For this review, take the finished solid that the model builds, in its own axes (mm). Face numbers are marked on the shaded views. A direction names the side the tool comes from. Give positions to 0.01 mm unless a question says otherwise; leave off trailing zeros. Loops run counter-clockwise (first coordinate to the right, second up) from the corner with the lowest first, then second, coordinate; pieces in that order, holes last. Notation, with made-up numbers: (17.25, 3) - (51.25, 3) arc R24 cw to (51.25, 39) - close; hole circle Ø8 at (42, -18.75). An arc over 180 degrees is marked (long way). Answer in a Markdown table with one row per item.
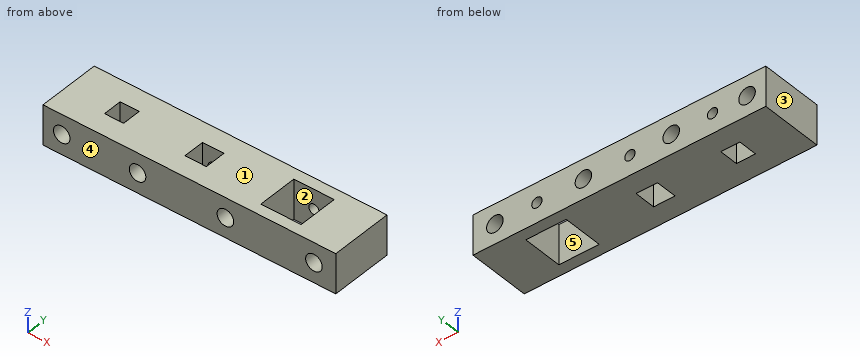
```python
from build123d import *

# Parameters (mm, degrees)
SKETCH1_W                       = 93.728
SKETCH1_H                       = 20
SKETCH1_W_2                     = 6.1
SKETCH1_H_2                     = 6.1
SKETCH1_W_3                     = 6.858
SKETCH1_H_3                     = 6.858
SKETCH1_W_4                     = 12.9
SKETCH1_H_4                     = 12.9
BOSS_EXTRUDE1_DEPTH             = 12.7
TAP_DRILL_FOR_M4X0_7_TAP1_D     = 3.3
TAP_DRILL_FOR_M4X0_7_TAP1_DEPTH = 6.95
M5_CLEARANCE_HOLE1_D            = 5.3


with BuildPart() as part:
    # Sketch1 → Boss-Extrude1 (new body)
    with BuildSketch(Plane.XY):
        with Locations((3.375, 0)):
            Rectangle(SKETCH1_W, SKETCH1_H)
        with Locations((-26.439, 0)):
            Rectangle(SKETCH1_W_2, SKETCH1_H_2, mode=Mode.SUBTRACT)
        Rectangle(SKETCH1_W_3, SKETCH1_H_3, mode=Mode.SUBTRACT)
        with Locations((29.789, 0)):
            Rectangle(SKETCH1_W_4, SKETCH1_H_4, mode=Mode.SUBTRACT)
    extrude(amount=BOSS_EXTRUDE1_DEPTH)

    # Tap Drill for M4x0.7 Tap1
    with Locations(Plane(origin=(-26.439, 10, 6.35), x_dir=(0, 0, 1), z_dir=(0, 1, 0))):
        with Locations((0, 0), (0, 26.439), (0, 56.228)):
            Hole(TAP_DRILL_FOR_M4X0_7_TAP1_D / 2, depth=TAP_DRILL_FOR_M4X0_7_TAP1_DEPTH)

    # M5 Clearance Hole1 (through all)
    with Locations(Plane(origin=(-37.489, 10, 6.35), x_dir=(0, 0, 1), z_dir=(0, 1, 0))):
        with Locations((0, 0), (0, 24.2695), (0, 52.3835), (0, 80.728)):
            Hole(M5_CLEARANCE_HOLE1_D / 2)


solid = part.part
```
1. For the marked faces 4 and 5, list the 3-axis set-ups (+Z, -Z, +X, -X, +Y, -Y) from which the entire face can be reached by the end or side of a thin tool; tool diameter is ignored.
Values:
| item | result |
|---|---|
| face 4 | +Z, -Z, +X, -X, -Y |
| face 5 | +Z, -Z |
2. Clearance check with a flat-ended pin moving along its axis: pin 1 (2.5 mm diameter, centred on x = 0, z = 6.35, fed in from +Y). State where the tip first meets the part, or that it passes through.
Values:
| item | result |
|---|---|
| pin 1 | stops at y = -3.43 |
3. Mouldability with a two-part tool opening along X and no side actions: class the marked faces 1, 2 and 3 as released by +X, released by -X, zero draft, split by the parting line, or undercut.
Values:
| item | result |
|---|---|
| face 1 | zero draft |
| face 2 | undercut |
| face 3 | released by -X |
4. We need section C-C, the plane y = -0.25. Give the boundary of the cut face in (x, z), and give its area (3 significant figures).
Values:
| item | result |
|---|---|
| outline | (-43.49, 0) - (-29.49, 0) - (-29.49, 12.7) - (-43.49, 12.7) - close; (-23.39, 0) - (-3.43, 0) - (-3.43, 12.7) - (-23.39, 12.7) - close; (3.43, 0) - (23.34, 0) - (23.34, 12.7) - (3.43, 12.7) - close; (36.24, 0) - (50.24, 0) - (50.24, 12.7) - (36.24, 12.7) - close; hole circle Ø5.3 at (-37.49, 6.35); hole circle Ø5.3 at (-13.22, 6.35); hole circle Ø5.3 at (14.89, 6.35); hole circle Ø5.3 at (43.24, 6.35) |
| area | 774 mm^2 |
5. We need section A-A, the plane z = 2.5. Give the boundary of the cut face in (x, y), and give its area (3 significant figures).
Values:
| item | result |
|---|---|
| outline | (-43.49, -10) - (50.24, -10) - (50.24, 10) - (-43.49, 10) - close; hole (-29.49, -3.05) - (-23.39, -3.05) - (-23.39, 3.05) - (-29.49, 3.05) - close; hole (-3.43, -3.43) - (3.43, -3.43) - (3.43, 3.43) - (-3.43, 3.43) - close; hole (23.34, -6.45) - (36.24, -6.45) - (36.24, 6.45) - (23.34, 6.45) - close |
| area | 1,620 mm^2 |
6. We need section B-B, the plane x = 44.5. Give the boundary of the cut face in (y, z).
Values:
| item | result |
|---|---|
| outline | (-10, 0) - (10, 0) - (10, 4.02) - (-10, 4.02) - close; (-10, 8.68) - (10, 8.68) - (10, 12.7) - (-10, 12.7) - close |
7. Wall thickness on line 1 (X direction, y = 0, z = 10.5); line 2 (Y direction, x = 3, z = 1.75); line 3 (Y direction, x = -24.5, z = 10): over which ranges is each line inside the solid? List them lowest first. Write a range as [from, to].
Values:
| item | result |
|---|---|
| line 1 | x = [-43.49, -29.49], [-23.39, -3.43], [3.43, 23.34], [36.24, 50.24] |
| line 2 | y = [-10, -3.43], [3.43, 10] |
| line 3 | y = [-10, -3.05], [3.05, 10] |
8. We need section D-D, the plane x = 0. Give the boundary of the cut face in (y, z).
Values:
| item | result |
|---|---|
| outline | (-10, 0) - (-3.43, 0) - (-3.43, 12.7) - (-10, 12.7) - close; (3.43, 0) - (10, 0) - (10, 4.7) - (3.43, 4.7) - close; (3.43, 8) - (10, 8) - (10, 12.7) - (3.43, 12.7) - close |
